```python
from build123d import *

# Parameters (mm, degrees)
SKETCH1_W           = 50
SKETCH1_H           = 40
BOSS_EXTRUDE1_DEPTH = 35
SKETCH2_W           = 42
SKETCH2_H           = 27
CUT_EXTRUDE1_DEPTH  = 59.736700622


with BuildPart() as part:
    # Sketch1 → Boss-Extrude1 (new body)
    with BuildSketch(Plane(origin=(0, 0, 0), x_dir=(1, 0, 0), z_dir=(0, 1, 0))):
        Rectangle(SKETCH1_W, SKETCH1_H)
    extrude(amount=BOSS_EXTRUDE1_DEPTH)

    # Sketch2 → Cut-Extrude1 (cut, through all)
    with BuildSketch(Plane.XY.offset(20)):
        with Locations((0, 17.5)):
            Rectangle(SKETCH2_W, SKETCH2_H)
    extrude(amount=-CUT_EXTRUDE1_DEPTH, mode=Mode.SUBTRACT)


solid = part.part
```
Check sheet for the modelled part. Datum: model origin and axes. Units: mm. A direction names the side the tool comes from. Give positions to 0.01 mm unless a question says otherwise; leave off trailing zeros. Order: outer loops, then holes, each group sorted by start corner. A loop starts at its lowest first (then second) coordinate and runs counter-clockwise, first axis right, second up. Notation, with made-up numbers: (46, 74) -> (58, 74) arc R20 ccw to (58, 113) -> close; hole circle Ø6 at (28.25, 58). An arc over 180 degrees is marked (long way). Use CSV: the item, a comma, the result in double quotes. Start each with the question number.
1) Mould release check, pull along X, two halves, no side actions. Record for faces 1 (the face through (0, 33, -20)), 2 (the face through (21, 17, 0)), 3 (the face through (25, 17, 0)): released by +X, released by -X, zero draft, split by the parting line, or undercut.
2) Sectioned sample at C-C, the plane x = -3. Record the boundary of the cut face in (y, z).
3) Material ranges on line 1 (X direction, y = 17, z = 14.5); line 2 (Y direction, x = 7.5, z = 11), recorded low to high. Write a range as from..to.
4) Set-up check for faces 4 (the face through (0, 31, 0)), 5 (the face through (-25, 17, 0)): record each of +Z, -Z, +X, -X, +Y, -Y from which the full face is reachable in a straight line by a thin tool's end or side.
5) Sectioned sample at A-A, the plane y = 27. Record the boundary of the cut face in (x, z), plus the area to 3 significant figures.
6) Sectioned sample at B-B, the plane z = -9.5. Record the boundary of the cut face in (x, y), plus the area to 3 significant figures.
Recorded:
1,face 1,"zero draft"
1,face 2,"undercut"
1,face 3,"released by +X"
2,outline,"(0, -20) -> (4, -20) -> (4, 20) -> (0, 20) -> close; (31, -20) -> (35, -20) -> (35, 20) -> (31, 20) -> close"
3,line 1,"-25..-21, 21..25"
3,line 2,"0..4, 31..35"
4,face 4,"+Z, -Z"
4,face 5,"+Z, -Z, -X, +Y, -Y"
5,outline,"(-25, -20) -> (-21, -20) -> (-21, 20) -> (-25, 20) -> close; (21, -20) -> (25, -20) -> (25, 20) -> (21, 20) -> close"
5,area,"320 mm2"
6,outline,"(-25, 0) -> (25, 0) -> (25, 35) -> (-25, 35) -> close; hole (-21, 4) -> (21, 4) -> (21, 31) -> (-21, 31) -> close"
6,area,"616 mm2"
